Can you work these out from the model? Positions are in its coordinate system, mm. Face numbers are marked on the shaded views. A direction names the side the tool comes from. Give positions to 0.01 mm unless a question says otherwise; leave off trailing zeros. Loops run counter-clockwise (first coordinate to the right, second up) from the corner with the lowest first, then second, coordinate; pieces in that order, holes last. Notation, with made-up numbers: (73.25, 15) - (122.25, 15) arc R25 cw to (122.25, 31) - close; hole circle Ø1 at (5.5, 51.25). An arc over 180 degrees is marked (long way). Answer as a JSON object with one key per item and string values.
```python
from build123d import *

# Parameters (mm, degrees)
EXTRUDE_1_DEPTH     = 10
SKETCH_2_R          = 2.500000000000002
SKETCH_2_R_2        = 2.5
CUT_EXTRUDE_1_DEPTH = 10
SKETCH_4_R          = 4.999999999999997
EXTRUDE_2_DEPTH     = 17.85
EXTRUDE_START       = -10
EXTRUDE_3_DEPTH     = 10
FILLET_1_R          = 2
CHAMFER_START       = 4
CHAMFER_1_OUTLINE_W = 8.394855713999998
CHAMFER_1_OUTLINE_H = 10
CHAMFER_1_DEPTH     = 3.536622653
SKETCH_6_R          = 2.500000000000002
CUT_EXTRUDE_2_DEPTH = 8
SKETCH_8_R          = 1.7500000000000036
CUT_EXTRUDE_4_DEPTH = 0.85
SKETCH_9_R          = 1.7499999999999967
CUT_EXTRUDE_5_DEPTH = 23.000000000000007
CUT_EXTRUDE_START   = -3
CUT_EXTRUDE_6_DEPTH = 4
FILLET_2_R          = 1
EXTRUDE_4_DEPTH     = 4
SKETCH_12_R         = 2.5
EXTRUDE_5_DEPTH     = 4


with BuildPart() as part:
    # 草图1 → 凸台-拉伸1 (new body)
    with BuildSketch(Plane.XY):
        with BuildLine():
            Line((0, 5), (50, 5.000000000000001))
            ThreePointArc((50, 5.000000000000001), (55, 0), (50, -4.999999999999997))
            Line((50, -4.999999999999997), (0, -5))
            ThreePointArc((0, -5), (-5, 6.1e-16), (0, 5))
        make_face()
    extrude(amount=EXTRUDE_1_DEPTH)

    # 草图2 → 切除-拉伸1 (cut)
    with BuildSketch(Plane.XY.offset(10)):
        with Locations((50, 0)):
            Circle(SKETCH_2_R)
        Circle(SKETCH_2_R_2)
    extrude(amount=-CUT_EXTRUDE_1_DEPTH, mode=Mode.SUBTRACT)

    # 草图4 → 凸台-拉伸2 (add)
    with BuildSketch(Plane.XY.offset(10)):
        with Locations(Location((50, 0, 0), (0, 0, 90))):
            Circle(SKETCH_4_R)
    extrude(amount=EXTRUDE_2_DEPTH)

    # 草图5 → 凸台-拉伸3 (add)
    with BuildSketch(Plane.XY.offset(10).offset(EXTRUDE_START)):
        with BuildLine():
            Line((-9.171946933133274, -2.4749524148530857), (-4.827340491122777, -1.3026065341332034))
            ThreePointArc((-4.827340491122777, -1.3026065341332034), (-3.0403097974823012, -3.9694478627805583), (5.411e-14, -5))
            Line((5.411e-14, -5), (1.028e-13, -9.5))
            ThreePointArc((1.028e-13, -9.5), (-5.7765886152163715, -7.541950939283059), (-9.171946933133274, -2.4749524148530857))
        make_face()
    extrude(amount=EXTRUDE_3_DEPTH)

    # 圆角1
    fillet_1_edges = [part.edges().sort_by_distance(p)[0] for p in [
        (1.028e-13, -9.5, 5),
    ]]
    fillet(fillet_1_edges, radius=FILLET_1_R)

    # 倒角1: read off the stored shape, not the designer's step
    # 倒角1 outline → 倒角1 (add)
    with BuildSketch(Plane(origin=(0, 0, 0), x_dir=(0.9076430982816491, 0.41974278569343915, 0), z_dir=(0.41974278569343915, -0.9076430982816494, 0)).offset(CHAMFER_START)):
        with Locations((0.18755170199999993, 5)):
            Rectangle(CHAMFER_1_OUTLINE_W, CHAMFER_1_OUTLINE_H)
    extrude(amount=CHAMFER_1_DEPTH)

    # 草图6 → 切除-拉伸2 (cut)
    with BuildSketch(Plane.XY.offset(27.85)):
        with Locations((50, 0)):
            Circle(SKETCH_6_R)
    extrude(amount=-CUT_EXTRUDE_2_DEPTH, mode=Mode.SUBTRACT)

    # 草图8 → 切除-拉伸4 (cut)
    with BuildSketch(Plane.XY.offset(19.849999999999998)):
        with Locations((50, 0)):
            Circle(SKETCH_8_R)
    extrude(amount=-CUT_EXTRUDE_4_DEPTH, mode=Mode.SUBTRACT)

    # 草图9 → 切除-拉伸5 (cut)
    with BuildSketch(Plane.XY.offset(19)):
        with Locations((50, 0)):
            Circle(SKETCH_9_R)
    extrude(amount=-CUT_EXTRUDE_5_DEPTH, mode=Mode.SUBTRACT)

    # 草图10 → 切除-拉伸6 (cut)
    with BuildSketch(Plane(origin=(0, 0, 0), x_dir=(-1, 0, 0), z_dir=(0, 0, -1)).offset(CUT_EXTRUDE_START)):
        with BuildLine():
            Line((9.171946933133274, -2.474952414853084), (4.827340491122777, -1.3026065341332034))
            ThreePointArc((4.827340491122777, -1.3026065341332034), (-4.327921927110574, 2.503815447039879), (3.535533905932719, -3.535533905932756))
            Line((3.535533905932719, -3.535533905932756), (6.717514421272165, -6.717514421272236))
            ThreePointArc((6.717514421272165, -6.717514421272236), (8.223051661510087, -4.757249349375768), (9.171946933133274, -2.474952414853084))
        make_face()
    extrude(amount=-CUT_EXTRUDE_6_DEPTH, mode=Mode.SUBTRACT)

    # 圆角2
    fillet_2_edges = [part.edges().sort_by_distance(p)[0] for p in [
        (-3.1e-16, 5, 5),
    ]]
    fillet(fillet_2_edges, radius=FILLET_2_R)

    # 草图11 → 凸台-拉伸4 (add)
    with BuildSketch(Plane.XY.offset(3)):
        with BuildLine():
            Line((-3.5355339059327213, -3.535533905932754), (-8.205808816608519, -4.78693029667969))
            ThreePointArc((-8.205808816608519, -4.78693029667969), (-7.523840965962772, -5.800156646065724), (-6.717514421272165, -6.717514421272236))
            Line((-6.717514421272165, -6.717514421272236), (-3.5355339059327213, -3.535533905932754))
        make_face()
    extrude(amount=EXTRUDE_4_DEPTH)

    # 草图12 → 凸台-拉伸5 (add)
    with BuildSketch(Plane.XY.offset(3)):
        with BuildLine():
            Line((-8.205808816608517, -4.786930296679689), (-3.5355339059327213, -3.535533905932754))
            ThreePointArc((-3.5355339059327213, -3.535533905932754), (3.435764551188546, -3.632564101126939), (3.726779962499649, 3.3333333333333344))
            ThreePointArc((3.726779962499649, 3.3333333333333344), (3.559265025824303, 4.408248290463864), (4.47213595499958, 5))
            Line((4.47213595499958, 5), (0, 5))
            ThreePointArc((0, 5), (-3.96944786278054, 3.0403097974823226), (-4.827340491122777, -1.3026065341332023))
            Line((-4.827340491122777, -1.3026065341332023), (-9.171946933133274, -2.474952414853084))
            ThreePointArc((-9.171946933133274, -2.474952414853084), (-8.765438332219034, -3.66293473106813), (-8.205808816608517, -4.786930296679689))
        make_face()
        Circle(SKETCH_12_R, mode=Mode.SUBTRACT)
    extrude(amount=EXTRUDE_5_DEPTH)


solid = part.part
```
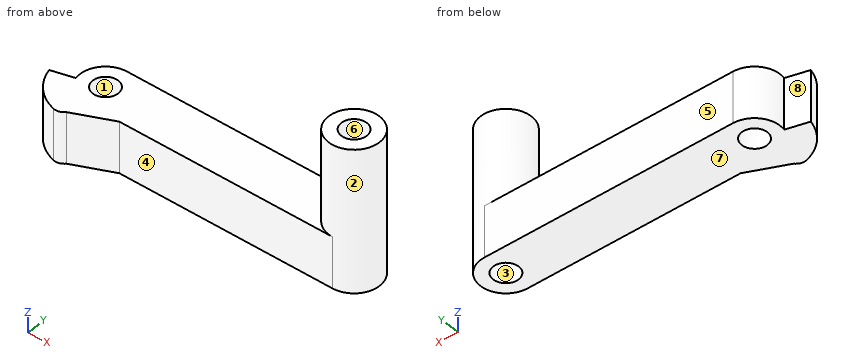
1) Which directions (+Z, -Z, +X, -X, +Y, -Y) give clear straight access to the entire face, cutting with the end or side of a thin tool? Please do the marked faces 1, 2, 3, 4 and 5.
Check sheet entries:
{"face 1": "+Z, -Z", "face 2": "+Z", "face 3": "-Z", "face 4": "+Z, -Z, +X, -Y", "face 5": "+Z, -Z, +X, -X, +Y"}
2) If we mould it in two halves opening along X, with no side actions, what happens to the marked faces 6, 7 and 8? For each: released by +X, released by -X, zero draft, split by the parting line, or undercut.
Check sheet entries:
{"face 6": "undercut", "face 7": "zero draft", "face 8": "released by -X"}
3) Imagine slicing it at A-A on y = 0. Write out the boundary of the cut face in (x, z), and give its area (3 significant figures).
Check sheet entries:
{"outline": "(-5, 0) - (-2.5, 0) - (-2.5, 10) - (-5, 10) - close; (2.5, 0) - (47.5, 0) - (47.5, 10) - (48.25, 10) - (48.25, 19.85) - (47.5, 19.85) - (47.5, 27.85) - (45, 27.85) - (45, 10) - (2.5, 10) - close; (51.75, 10) - (52.5, 10) - (52.5, 0) - (55, 0) - (55, 27.85) - (52.5, 27.85) - (52.5, 19.85) - (51.75, 19.85) - close", "area": "604 mm2"}
4) I'm going to push flat-ended pins straight in: P1, Ø5, axis at x = 33.5, y = 1.5, coming from the +Z side; P2, Ø5, axis at x = 37, z = 6, coming from the -Y side; P3, Ø2, axis at y = -7, z = 7, coming from the -X side; P4, Ø3, axis at x = 44, y = -7, coming from the +Z side. Where does each tip first touch, or does it pass through?
Check sheet entries:
{"P1": "z = 10", "P2": "y = -5", "P3": "x = -7.37", "P4": "through"}
5) Imagine slicing it at C-C on x = 15. Write out the boundary of the cut face in (y, z).
Check sheet entries:
{"outline": "(-5, 0) - (5, 0) - (5, 10) - (-5, 10) - close"}
6) I need wall thicknesses on L1, parallel to Y at x = 50, z = 12.5; L2, parallel to Y at x = 50, z = 23; L3, parallel to X at y = -1, z = 4.25. Which ranges of each line are inside material? Lowest first, please.
Check sheet entries:
{"L1": "-5 to -1.75, 1.75 to 5", "L2": "-5 to -2.5, 2.5 to 5", "L3": "-4.9 to -2.29, 2.29 to 47.71, 52.29 to 54.9"}
7) Imagine slicing it at B-B on z = 26. Write out the boundary of the cut face in (x, y), and give its area (3 significant figures).
Check sheet entries:
{"outline": "circle Ø10 at (50, 0); hole circle Ø5 at (50, 0)", "area": "58.9 mm2"}
8) Imagine slicing it at D-D on y = 3.5. Write out the boundary of the cut face in (x, z), and give its area (3 significant figures).
Check sheet entries:
{"outline": "(-3.57, 0) - (53.57, 0) - (53.57, 27.85) - (46.43, 27.85) - (46.43, 10) - (-3.57, 10) - close", "area": "699 mm2"}
